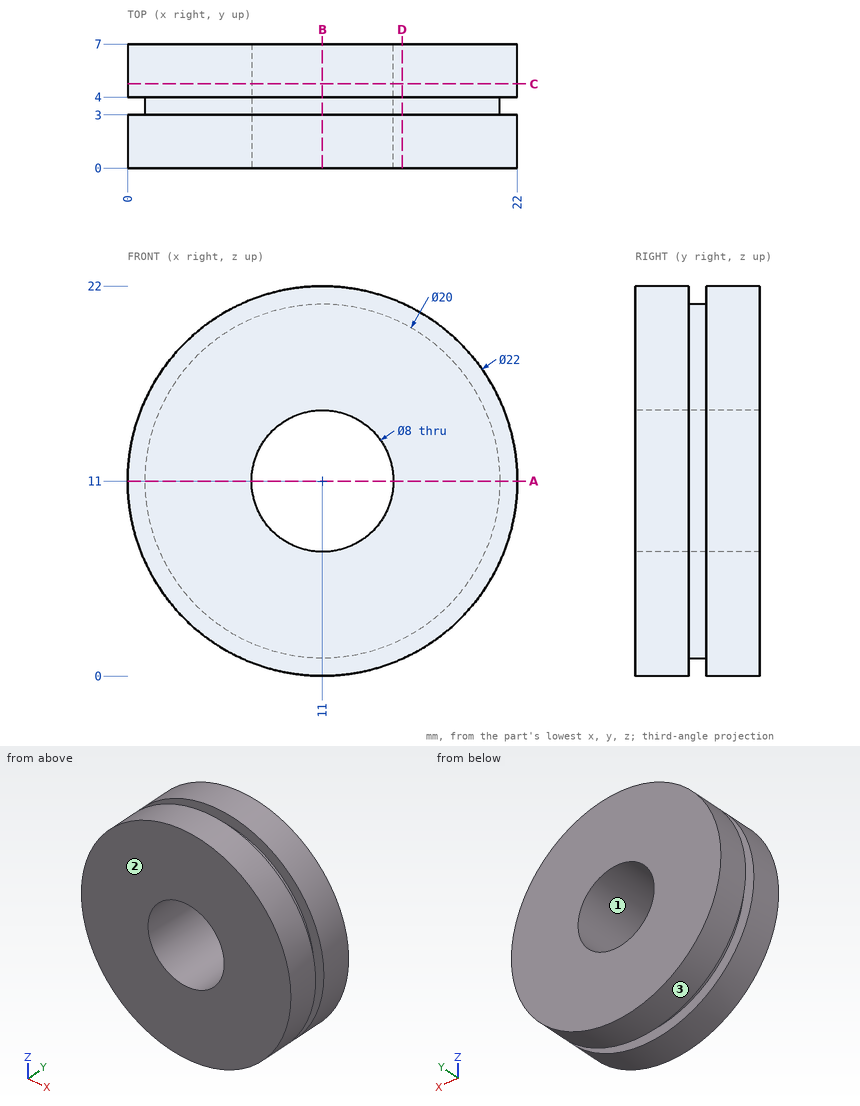
Could you check a few things on this drawing? It's one solid part, dimensions in mm from its lowest x, y, z. Coordinates: 2 decimals unless noted, no trailing zeros. Loops run counter-clockwise (first coordinate to the right, second up) from the corner with the lowest first, then second, coordinate; pieces in that order, holes last. Notation, with made-up numbers: (22.25, 67.25) - (42.25, 67.25) arc R28 ccw to (42.25, 98.25) - close; hole circle Ø9 at (40, 15). An arc over 180 degrees is marked (long way). Return JSON: item names as keys, results as strings. Group by question number.
Item 1: If we section it at C-C on y = 4.75: Write out the boundary of the cut face in (x, z), and give its area (3 significant figures).
Item 2: If we section it at D-D on x = 15.5: Write out the boundary of the cut face in (y, z).
Item 3: Will these pins go through, and if not, where does the flat tip stop? P1, Ø1, axis at y = 1.5, z = 19, coming from the +X side; P2, Ø1.5, axis at y = 1.5, z = 10, coming from the +X side.
Item 4: I need wall thicknesses on line 1 (Z direction, x = 11, y = 2.75); line 2 (Y direction, x = 19, z = 17.5). Which ranges of each line are inside material? Lowest first, please. Write a range as from..to.
Item 5: We'd pull the mould along Z, two halves only. Please class the marked faces 1, 2 and 3: +Z half, -Z half, draft (parallel to the pull), parting line (faces both ways), or undercut.
Item 6: If we section it at B-B on x = 11: Write out the boundary of the cut face in (y, z), and give its area (3 significant figures).
Item 7: If we section it at A-A on z = 11: Write out the boundary of the cut face in (x, y).
Calculated:
{
 "1": {"outline": "circle Ø22 at (11, 11); hole circle Ø8 at (11, 11)", "area": "330 mm^2"},
 "2": {"outline": "(0, 0.96) - (3, 0.96) - (3, 2.07) - (4, 2.07) - (4, 0.96) - (7, 0.96) - (7, 21.04) - (4, 21.04) - (4, 19.93) - (3, 19.93) - (3, 21.04) - (0, 21.04) - close"},
 "3": {"P1": "stops at x = 19.05", "P2": "stops at x = 22"},
 "4": {"line 1": "z = 0..7, 15..22", "line 2": "y = 0..3, 4..7"},
 "5": {"face 1": "undercut", "face 2": "draft", "face 3": "parting line"},
 "6": {"outline": "(0, 0) - (3, 0) - (3, 1) - (4, 1) - (4, 0) - (7, 0) - (7, 7) - (0, 7) - close; (0, 15) - (7, 15) - (7, 22) - (4, 22) - (4, 21) - (3, 21) - (3, 22) - (0, 22) - close", "area": "96.0 mm^2"},
 "7": {"outline": "(0, 0) - (7, 0) - (7, 7) - (0, 7) - (0, 4) - (1, 4) - (1, 3) - (0, 3) - close; (15, 0) - (22, 0) - (22, 3) - (21, 3) - (21, 4) - (22, 4) - (22, 7) - (15, 7) - close"}
}
